The model under review builds one solid part; all positions refer to its coordinate system, in mm. Face numbers are marked on the shaded views. A direction names the side the tool comes from. Coordinates: 2 decimals unless noted, no trailing zeros. Loops run counter-clockwise (first coordinate to the right, second up) from the corner with the lowest first, then second, coordinate; pieces in that order, holes last. Notation, with made-up numbers: (-4, -27.75) - (15, -27.75) arc R18 ccw to (15, -18.75) - close; hole circle Ø4 at (51.5, 20.5). An arc over 180 degrees is marked (long way). Use a Markdown table: item, result. Add a question column.
1) To check wall thickness, follow L1, parallel to Y at x = -3.75, z = 122.25; L2, parallel to Z at x = 0, y = -13.5; L3, parallel to Y at x = -5, z = 120.5. State the ranges of each line that lie inside material, in increasing order. Write a range as [from, to].
2) Add section A-A, the plane z = 122. Give the boundary of the cut face in (x, y), and give its area (3 significant figures).
3) For the marked faces 1, 2 and 3, list the 3-axis set-ups (+Z, -Z, +X, -X, +Y, -Y) from which the entire face can be reached by the end or side of a thin tool; tool diameter is ignored.
4) The part is to be moulded in two halves that separate along Y. For the marked faces 4, 5 and 6, say which applies: pulls with the +Y half, pulls with the -Y half, needs draft (parallel to the pull), parting line crosses it, or undercut.
5) Add section B-B, the plane y = -21. Give the boundary of the cut face in (x, z).
6) Clearance check with flat-ended pins moving along their axes: pin 1 (2 mm diameter, centred on y = -10.5, z = 126, fed in from -X); pin 2 (1.5 mm diameter, centred on y = -16, z = 114, fed in from -X). State where each tip first meets the part, or that it passes through.
7) Add section C-C, the plane y = -7. Give the boundary of the cut face in (x, z), and give its area (3 significant figures).
```python
from build123d import *

# Parameters (mm, degrees)
PAD001002_DEPTH      = 17
PAD001002_DEPTH_BACK = 10
PAD001003_DEPTH      = 4.5
SKETCH006_W          = 10
SKETCH006_H          = 13
POCKET002_DEPTH      = 10.440828
CHAMFER_SIZE         = 0.6
PAD001004_DEPTH      = 13


with BuildPart() as part:
    # Sketch004 → Pad001002 (new body, two sides)
    with BuildSketch(Plane.XZ.offset(15)) as pad001002_sk:
        with BuildLine():
            ThreePointArc((-5.219914, 117.25), (0, 114.1), (5.219914, 117.25))
            Line((5.219914, 117.25), (5.219914, 122.75))
            ThreePointArc((5.219914, 122.75), (0, 125.9), (-5.219914, 122.75))
            Line((-5.219914, 122.75), (-5.219914, 117.25))
        make_face()
    extrude(amount=PAD001002_DEPTH)
    extrude(pad001002_sk.sketch, amount=-PAD001002_DEPTH_BACK)

    # Sketch005 → Pad001003 (new body)
    with BuildSketch(Plane(origin=(0, -5, 0), x_dir=(1, 0, 0), z_dir=(0, 1, 0))):
        with BuildLine():
            ThreePointArc((5.219914, -114.070202), (0, -112.1), (-5.219914, -114.070202))
            Line((-5.219914, -125.929798), (-5.219914, -114.070202))
            ThreePointArc((-5.219914, -125.929798), (0, -127.9), (5.219914, -125.929798))
            Line((5.219914, -114.070202), (5.219914, -125.929798))
        make_face()
    extrude(amount=PAD001003_DEPTH)

    # Sketch006 → Pocket002 (cut, through all)
    with BuildSketch(Plane(origin=(5.219914, -15, 0), x_dir=(0, 0, 1), z_dir=(1, 0, 0))):
        with Locations((124.75, 8.5)):
            Rectangle(SKETCH006_W, SKETCH006_H)
    extrude(amount=-POCKET002_DEPTH, mode=Mode.SUBTRACT)

    # Chamfer
    chamfer_edges = [part.edges().sort_by_distance(p)[0] for p in [
        (0, -32, 114.1),
        (5.219914, -32, 120),
        (0, -32, 125.9),
        (-5.219914, -32, 120),
    ]]
    chamfer(chamfer_edges, length=CHAMFER_SIZE)

    # Sketch007 → Pad001004 (new body)
    with BuildSketch(Plane.XZ.offset(17)):
        with BuildLine():
            ThreePointArc((5.219914, 119.75), (0, 122.9), (-5.219914, 119.75))
            Line((-5.219914, 119.75), (5.219914, 119.75))
        make_face()
    extrude(amount=PAD001004_DEPTH)


solid = part.part
```
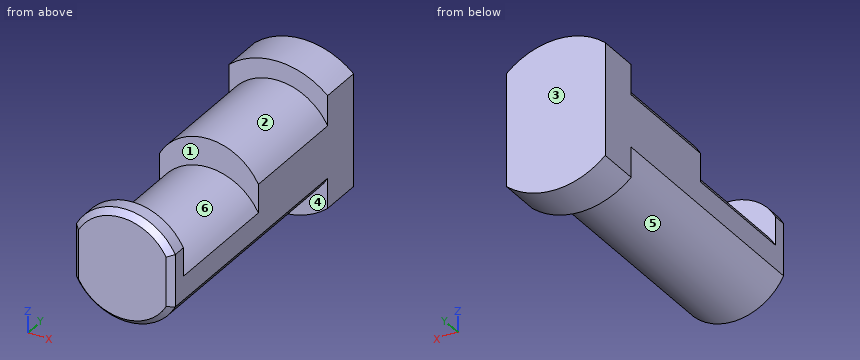
From the geometry:
| question | item | result |
|---|---|---|
| 1 | L1 | y = [-32, -30], [-17, -0.5] |
| 1 | L2 | z = [114.1, 125.9] |
| 1 | L3 | y = [-31.62, -30], [-17, -0.5] |
| 2 | outline | (-5.22, -31.4) - (-4.62, -32) - (4.62, -32) - (5.22, -31.4) - (5.22, -30) - (3.13, -30) - (3.13, -17) - (5.22, -17) - (5.22, -0.5) - (-5.22, -0.5) - (-5.22, -17) - (-3.13, -17) - (-3.13, -30) - (-5.22, -30) - close |
| 2 | area | 274 mm^2 |
| 3 | face 1 | +Z |
| 3 | face 2 | +Z, -Y |
| 3 | face 3 | +Z, -Z, +X, -X, +Y |
| 4 | face 4 | pulls with the -Y half |
| 4 | face 5 | needs draft |
| 4 | face 6 | undercut |
| 5 | outline | (-5.22, 117.25) arc R5.9 ccw to (5.22, 117.25) - (5.22, 119.75) arc R5.9 ccw to (-5.22, 119.75) - close |
| 6 | pin 1 | stops at x = -3.13 |
| 6 | pin 2 | stops at x = -2.69 |
| 7 | outline | (-5.22, 117.25) arc R5.9 ccw to (5.22, 117.25) - (5.22, 122.75) arc R5.9 ccw to (-5.22, 122.75) - close |
| 7 | area | 104 mm^2 |
